Input: part model. Units: mm. Frame: model coordinates. Give positions to 0.01 mm unless a question says otherwise; leave off trailing zeros. Order: outer loops, then holes, each group sorted by start corner. A loop starts at its lowest first (then second) coordinate and runs counter-clockwise, first axis right, second up. Notation, with made-up numbers: (-4, 67.25) - (41, 67.25) arc R14 ccw to (41, 83.25) - close; hole circle Ø10 at (63, -32). An arc over 180 degrees is marked (long way). Use a Markdown table: item, result.
from build123d import *

# Parameters (mm, degrees)
SKETCH1_R                        = 4.951729289
BOSS_EXTRUDE3_DEPTH              = 3
BOSS_EXTRUDE4_DEPTH              = 68
SKETCH5_R                        = 4.5
CUT_EXTRUDE1_DEPTH               = 68
SKETCH11_W                       = 45.01572081
SKETCH11_H                       = 71
CUT_EXTRUDE3_DEPTH               = 2.5
SKETCH12_R                       = 13
BOSS_EXTRUDE7_DEPTH              = 3
SKETCH13_W                       = 45.01572081
SKETCH13_H                       = 71
CUT_EXTRUDE4_DEPTH               = 13
SKETCH14_W                       = 45.01572081
SKETCH14_H                       = 71
BOSS_EXTRUDE8_DEPTH              = 3
SKETCH15_R                       = 1.5
BOSS_EXTRUDE11_DEPTH             = 56.52620135
SKETCH16_R                       = 9
SKETCH16_R_2                     = 4.15
BOSS_EXTRUDE12_DEPTH             = 2
BOSS_EXTRUDE12_DIRECTION_2_REACH = 85.837
SKETCH17_R                       = 9
SKETCH17_R_2                     = 1
BOSS_EXTRUDE13_DEPTH             = 2
SKETCH18_R                       = 13
SKETCH18_R_2                     = 1
BOSS_EXTRUDE14_DEPTH             = 3
SKETCH19_R                       = 1.5
SKETCH19_R_2                     = 1
BOSS_EXTRUDE15_DEPTH             = 56.52620135
CUT_EXTRUDE9_DEPTH               = 43.52620135
SKETCH27_R                       = 10
SKETCH27_R_2                     = 1
CUT_EXTRUDE12_DEPTH              = 10
SKETCH28_R                       = 4.15
CUT_EXTRUDE13_DEPTH              = 73
SKETCH29_R                       = 4.5
SKETCH29_R_2                     = 4.15
CUT_EXTRUDE14_DEPTH              = 73
SKETCH30_R                       = 9
CUT_EXTRUDE15_DEPTH              = 4
SKETCH31_R                       = 10.2
CUT_EXTRUDE17_DEPTH              = 3
CUT_EXTRUDE18_DEPTH              = 197
SKETCH33_W                       = 14.992341928
SKETCH33_H                       = 71
BOSS_EXTRUDE16_DEPTH             = 1
SKETCH34_W                       = 14.992341928
SKETCH34_H                       = 71
BOSS_EXTRUDE17_DEPTH             = 1


with BuildPart() as part:
    # Sketch1 → Boss-Extrude3 (new body)
    with BuildSketch(Plane(origin=(0, 0, 0), x_dir=(1, 0, 0), z_dir=(0, 1, 0))):
        Polygon((-55.988214466, 21.072670098), (19.011785534, 23.055317054), (20.201373708, -21.944682946), (-54.798626292, -23.927329902), align=None)
        with Locations(Location((-17.893420379, -0.436006424, 0), (0, 0, 270))):
            Circle(SKETCH1_R, mode=Mode.SUBTRACT)
    extrude(amount=BOSS_EXTRUDE3_DEPTH)

    # Sketch4 → Boss-Extrude4 (add)
    with BuildSketch(Plane(origin=(0, 3, 0), x_dir=(1, 0, 0), z_dir=(0, 1, 0))):
        Polygon((-54.798626292, -23.927329902), (20.201373708, -21.944682946), (19.011785534, 23.055317054), (-55.988214466, 21.072670098), align=None)
        Polygon((-52.365564518, -21.362137824), (17.636181629, -19.511621172), (16.578723759, 20.490124975), (-53.423022387, 18.639608323), align=None, mode=Mode.SUBTRACT)
    extrude(amount=BOSS_EXTRUDE4_DEPTH)

    # Sketch5 → Cut-Extrude1 (cut)
    with BuildSketch(Plane(origin=(19.607557344, 0, -0.518331518), x_dir=(-0.026426060768931774, 0, -0.9996507706755579), z_dir=(0.999650770675558, 0, -0.026426060768931777))):
        with Locations((0.036998456, 35.5)):
            Circle(SKETCH5_R)
        with BuildLine():
            ThreePointArc((-17.463001544, 29.25), (-19.213001544, 27.5), (-17.463001544, 25.75))
            ThreePointArc((-17.463001544, 25.75), (-15.713001544, 27.5), (-17.463001544, 29.25))
        make_face()
        with BuildLine():
            ThreePointArc((17.536998456, 25.75), (19.286998456, 27.5), (17.536998456, 29.25))
            ThreePointArc((17.536998456, 29.25), (15.786998456, 27.5), (17.536998456, 25.75))
        make_face()
    extrude(amount=-CUT_EXTRUDE1_DEPTH, mode=Mode.SUBTRACT)

    # Sketch11 → Cut-Extrude3 (cut)
    with BuildSketch(Plane(origin=(19.607557344, 0, -0.518331518), x_dir=(-0.026426060768931756, 0, -0.9996507706755579), z_dir=(0.999650770675558, 0, -0.02642606076893176))):
        with Locations((0.036998456, 35.5)):
            Rectangle(SKETCH11_W, SKETCH11_H)
    extrude(amount=-CUT_EXTRUDE3_DEPTH, mode=Mode.SUBTRACT)

    # Sketch12 → Boss-Extrude7 (add)
    with BuildSketch(Plane(origin=(0, 71, 0), x_dir=(1, 0, 0), z_dir=(0, 1, 0))):
        Polygon((17.636181629, -19.511621172), (16.578723759, 20.490124975), (-53.423022387, 18.639608323), (-52.365564518, -21.362137824), align=None)
        with Locations(Location((-17.893420379, -0.436006424, 0), (0, 0, 270))):
            Circle(SKETCH12_R, mode=Mode.SUBTRACT)
    extrude(amount=-BOSS_EXTRUDE7_DEPTH)

    # Sketch13 → Cut-Extrude4 (cut)
    with BuildSketch(Plane(origin=(-55.392442656, 0, 1.464315438), x_dir=(0.02642606076893168, 0, 0.9996507706755579), z_dir=(-0.999650770675558, 0, 0.026426060768931683))):
        with Locations((-0.036998456, 35.5)):
            Rectangle(SKETCH13_W, SKETCH13_H)
    extrude(amount=-CUT_EXTRUDE4_DEPTH, mode=Mode.SUBTRACT)

    # Sketch14 → Boss-Extrude8 (add)
    with BuildSketch(Plane(origin=(-42.396982637, 0, 1.120776648), x_dir=(0.026426060768931694, 0, 0.9996507706755579), z_dir=(-0.999650770675558, 0, 0.026426060768931697))):
        with Locations((-0.036998456, 35.5)):
            Rectangle(SKETCH14_W, SKETCH14_H)
    extrude(amount=-BOSS_EXTRUDE8_DEPTH)

    # Sketch15 → Boss-Extrude11 (add)
    with BuildSketch(Plane(origin=(17.108430418, 0, -0.452266367), x_dir=(-0.02642606076893177, 0, -0.9996507706755579), z_dir=(0.999650770675558, 0, -0.026426060768931774))):
        with BuildLine():
            ThreePointArc((20.044858861, 9.08994731), (14.741558002, 8.303300859), (13.954911551, 3))
            Line((13.954911551, 3), (20.044858861, 3))
            Line((20.044858861, 3), (20.044858861, 9.08994731))
        make_face()
        with Locations((17.923538517, 5.121320344)):
            Circle(SKETCH15_R, mode=Mode.SUBTRACT)
        with BuildLine():
            Line((-19.970861949, 9.08994731), (-19.970861949, 3))
            Line((-19.970861949, 3), (-13.880914639, 3))
            ThreePointArc((-13.880914639, 3), (-14.66756109, 8.303300859), (-19.970861949, 9.08994731))
        make_face()
        with Locations((-17.849541605, 5.121320344)):
            Circle(SKETCH15_R, mode=Mode.SUBTRACT)
        with BuildLine():
            Line((20.044858861, 68), (13.954911551, 68))
            ThreePointArc((13.954911551, 68), (14.741558002, 62.696699141), (20.044858861, 61.91005269))
            Line((20.044858861, 61.91005269), (20.044858861, 68))
        make_face()
        with Locations((17.923538517, 65.878679656)):
            Circle(SKETCH15_R, mode=Mode.SUBTRACT)
        with BuildLine():
            Line((-19.970861949, 68), (-19.970861949, 61.91005269))
            ThreePointArc((-19.970861949, 61.91005269), (-14.66756109, 62.696699141), (-13.880914639, 68))
            Line((-13.880914639, 68), (-19.970861949, 68))
        make_face()
        with Locations((-17.849541605, 65.878679656)):
            Circle(SKETCH15_R, mode=Mode.SUBTRACT)
    extrude(amount=-BOSS_EXTRUDE11_DEPTH)

    # Sketch16 → Boss-Extrude12 (add)
    with BuildSketch(Plane(origin=(0, 3, 0), x_dir=(1, 0, 0), z_dir=(0, 1, 0))):
        with Locations(Location((-17.893420379, -0.436006424, 0), (0, 0, 270))):
            Circle(SKETCH16_R)
        with Locations(Location((-17.893420379, -0.436006424, 0), (0, 0, 270))):
            Circle(SKETCH16_R_2, mode=Mode.SUBTRACT)
    extrude(amount=BOSS_EXTRUDE12_DEPTH)

    # Boss-Extrude12 direction 2: up to this face of the body (flat: up to its plane)
    boss_extrude12_direction_2_end = Plane(part.part.faces().sort_by_distance((-12.489919849, 0, 0.293163306))[0])
    # Sketch16 → Boss-Extrude12 direction 2 (add, up to the picked face)
    with BuildSketch(Plane(origin=(0, 3, 0), x_dir=(1, 0, 0), z_dir=(0, 1, 0)), mode=Mode.PRIVATE) as boss_extrude12_direction_2_sk1:
        with Locations(Location((-17.893420379, -0.436006424, 0), (0, 0, 270))):
            Circle(SKETCH16_R)
        with Locations(Location((-17.893420379, -0.436006424, 0), (0, 0, 270))):
            Circle(SKETCH16_R_2, mode=Mode.SUBTRACT)
    boss_extrude12_direction_2_tool1 = split(extrude(boss_extrude12_direction_2_sk1.sketch, amount=-BOSS_EXTRUDE12_DIRECTION_2_REACH, mode=Mode.PRIVATE), bisect_by=boss_extrude12_direction_2_end, keep=Keep.BOTH, mode=Mode.PRIVATE)
    add(boss_extrude12_direction_2_tool1.solids().sort_by(Axis((-17.89342, 3, -8.309435), (0, -1, 0)))[0])

    # Sketch17 → Boss-Extrude13 (add)
    with BuildSketch(Plane(origin=(0, 5, 0), x_dir=(1, 0, 0), z_dir=(0, 1, 0))):
        with Locations(Location((-17.893420379, -0.436006424, 0), (0, 0, 270))):
            Circle(SKETCH17_R)
        with Locations(Location((-17.893420379, -0.436006424, 0), (0, 0, 270))):
            Circle(SKETCH17_R_2, mode=Mode.SUBTRACT)
    extrude(amount=BOSS_EXTRUDE13_DEPTH)

    # Sketch18 → Boss-Extrude14 (add)
    with BuildSketch(Plane(origin=(0, 71, 0), x_dir=(1, 0, 0), z_dir=(0, 1, 0))):
        with Locations((-17.893420379, -0.436006424)):
            Circle(SKETCH18_R)
        with Locations(Location((-17.893420379, -0.436006424, 0), (0, 0, 270))):
            Circle(SKETCH18_R_2, mode=Mode.SUBTRACT)
    extrude(amount=-BOSS_EXTRUDE14_DEPTH)

    # Sketch19 → Boss-Extrude15 (add)
    with BuildSketch(Plane(origin=(17.108430418, 0, -0.452266367), x_dir=(-0.02642606076893177, 0, -0.9996507706755579), z_dir=(0.999650770675558, 0, -0.026426060768931774))):
        with Locations((-17.849541605, 5.121320344)):
            Circle(SKETCH19_R)
        with Locations((-17.849541605, 5.121320344)):
            Circle(SKETCH19_R_2, mode=Mode.SUBTRACT)
        with Locations((17.923538517, 5.121320344)):
            Circle(SKETCH19_R)
        with Locations((17.923538517, 5.121320344)):
            Circle(SKETCH19_R_2, mode=Mode.SUBTRACT)
        with Locations((-17.849541605, 65.878679656)):
            Circle(SKETCH19_R)
        with Locations((-17.849541605, 65.878679656)):
            Circle(SKETCH19_R_2, mode=Mode.SUBTRACT)
        with Locations((17.923538517, 65.878679656)):
            Circle(SKETCH19_R)
        with Locations((17.923538517, 65.878679656)):
            Circle(SKETCH19_R_2, mode=Mode.SUBTRACT)
    extrude(amount=-BOSS_EXTRUDE15_DEPTH)

    # Sketch23 → Cut-Extrude9 (cut)
    with BuildSketch(Plane(origin=(4.112970399, 0, -0.108727577), x_dir=(-0.02642606076893177, 0, -0.9996507706755579), z_dir=(0.999650770675558, 0, -0.026426060768931774))):
        Polygon((-19.970861949, 68), (-19.970861949, 9.08994731), (-19.970861949, 3), (-13.880914639, 3), (-8.963001544, 3), (-8.963001544, 7), (9.036998456, 7), (9.036998456, 3), (20.044858861, 3), (20.044858861, 9.08994731), (20.044858861, 68), (-13.880914639, 68), align=None)
    extrude(amount=-CUT_EXTRUDE9_DEPTH, mode=Mode.SUBTRACT)

    # Sketch27 → Cut-Extrude12 (cut)
    with BuildSketch(Plane(origin=(0, 71, 0), x_dir=(1, 0, 0), z_dir=(0, 1, 0))):
        with Locations(Location((-17.893420379, -0.436006424, 0), (0, 0, 270))):
            Circle(SKETCH27_R)
        with Locations(Location((-17.893420379, -0.436006424, 0), (0, 0, 270))):
            Circle(SKETCH27_R_2, mode=Mode.SUBTRACT)
    extrude(amount=-CUT_EXTRUDE12_DEPTH, mode=Mode.SUBTRACT)

    # Sketch28 → Cut-Extrude13 (cut)
    with BuildSketch(Plane.XZ):
        with Locations(Location((-17.893420379, 0.436006424, 0), (0, 0, 90))):
            Circle(SKETCH28_R)
    extrude(amount=-CUT_EXTRUDE13_DEPTH, mode=Mode.SUBTRACT)

    # Sketch29 → Cut-Extrude14 (cut)
    with BuildSketch(Plane.XZ):
        with Locations(Location((-17.893420379, 0.436006424, 0), (0, 0, 270))):
            Circle(SKETCH29_R)
        with Locations((-17.893420379, 0.436006424)):
            Circle(SKETCH29_R_2, mode=Mode.SUBTRACT)
    extrude(amount=-CUT_EXTRUDE14_DEPTH, mode=Mode.SUBTRACT)

    # Sketch30 → Cut-Extrude15 (cut)
    with BuildSketch(Plane(origin=(0, 7, 0), x_dir=(1, 0, 0), z_dir=(0, 1, 0))):
        with Locations((-17.893420379, -0.436006424)):
            Circle(SKETCH30_R)
    extrude(amount=-CUT_EXTRUDE15_DEPTH, mode=Mode.SUBTRACT)

    # Sketch31 → Cut-Extrude17 (cut)
    with BuildSketch(Plane(origin=(0, 71, 0), x_dir=(1, 0, 0), z_dir=(0, 1, 0))):
        with Locations(Location((-17.893420379, -0.436006424, 0), (0, 0, 270))):
            Circle(SKETCH31_R)
    extrude(amount=-CUT_EXTRUDE17_DEPTH, mode=Mode.SUBTRACT)

    # Sketch32 → Cut-Extrude18 (cut)
    with BuildSketch(Plane(origin=(0, 71, 0), x_dir=(1, 0, 0), z_dir=(0, 1, 0))):
        Polygon((-42.992754447, 21.416208888), (-42.703678037, 10.480963623), (-32.74415639, 21.687133577), align=None)
        Polygon((-31.554568217, -23.312866423), (-42.092242683, -12.648545848), (-41.803166274, -23.583791112), align=None)
    extrude(amount=-CUT_EXTRUDE18_DEPTH, mode=Mode.SUBTRACT)

    # Sketch33 → Boss-Extrude16 (add)
    with BuildSketch(Plane(origin=(-27.621364057, 0, 27.293341448), x_dir=(0.7028704732937463, 0, 0.7113178598712571), z_dir=(-0.7113178598712571, 0, 0.7028704732937463))):
        with Locations((-13.09208701, 35.5)):
            Rectangle(SKETCH33_W, SKETCH33_H)
    extrude(amount=-BOSS_EXTRUDE16_DEPTH)

    # Sketch34 → Boss-Extrude17 (add)
    with BuildSketch(Plane(origin=(-29.062615571, 0, -25.829498399), x_dir=(-0.6643072639922937, 0, 0.7474596035954538), z_dir=(-0.7474596035954538, 0, -0.6643072639922937))):
        with Locations((13.038095641, 35.5)):
            Rectangle(SKETCH34_W, SKETCH34_H)
    extrude(amount=-BOSS_EXTRUDE17_DEPTH)


solid = part.part
1. Section query B-B (x = -4.5). Return loops of the section in (y, z), then the cut area to 3 significant figures.
Response:
| item | result |
|---|---|
| outline | (0, -22.43) - (71, -22.43) - (71, 22.6) - (0, 22.6) - close; hole (3, -19.93) - (68, -19.93) - (68, 20.1) - (3, 20.1) - close |
| area | 595 mm^2 |
2. Pin query (flat end, axial travel): pin 1 (8 mm diameter, centred on y = 57, z = -7.5, fed in from +X); pin 2 (1 mm diameter, centred on y = 35, z = 18.5, fed in from +X); pin 3 (3 mm diameter, centred on x = -8.5, y = 59, fed in from -Z); pin 4 (1.5 mm diameter, centred on x = -27, z = -4, fed in from +Y). Return the tip coordinate at first contact, or that it passes through.
Response:
| item | result |
|---|---|
| pin 1 | stops at x = -39.52 |
| pin 2 | stops at x = -34.41 |
| pin 3 | stops at z = -22.37 |
| pin 4 | stops at y = 71 |
3. Mould query, pull axis Y, two halves, no side actions, for faces 1 (the face through (-35.865, 35.955, 17.528)), 2 (the face through (-22.286, 1.479, 1.412)). Classes: pulls with the +Y half, pulls with the -Y half, needs draft (parallel to the pull), parting line crosses it, or undercut.
Response:
| item | result |
|---|---|
| face 1 | undercut |
| face 2 | needs draft |
4. Section query A-A (z = 2). Return loops of the section in (x, y), then the cut area to 3 significant figures.
Response:
| item | result |
|---|---|
| outline | (-42.37, 0) - (-22.11, 0) - (-22.11, 3) - (-39.37, 3) - (-39.37, 68) - (-27.97, 68) - (-27.97, 71) - (-42.37, 71) - close; (-13.67, 0) - (17.17, 0) - (17.17, 3) - (-13.67, 3) - close; (-7.81, 68) - (17.17, 68) - (17.17, 71) - (-7.81, 71) - close |
| area | 467 mm^2 |
5. Material intervals for line 1 along Y through (x, z) = (-13.5, 19); line 2 along Y through (x, z) = (15.5, -18.5); line 3 along Z through (x, y) = (14.5, 27.5), sorted ascending.
Response:
| item | result |
|---|---|
| line 1 | y = 0 to 3, 68 to 71 |
| line 2 | y = 0 to 4.13, 6.11 to 9.62, 61.38 to 64.89, 66.87 to 71 |
| line 3 | z = -22.94 to -20.44, 19.59 to 22.1 |
6. Section query C-C (z = -5). Return loops of the section in (x, y).
Response:
| item | result |
|---|---|
| outline | (-42.56, 0) - (16.99, 0) - (16.99, 3) - (-39.56, 3) - (-39.56, 68) - (-26.52, 68) - (-26.52, 71) - (-42.56, 71) - close; (-9.26, 68) - (16.99, 68) - (16.99, 71) - (-9.26, 71) - close |
7. Section query D-D (y = 13.5). Return loops of the section in (x, z), then the cut area to 3 significant figures.
Response:
| item | result |
|---|---|
| outline | (-42.7, -10.48) - (-32.74, -21.69) - (16.51, -22.99) - (16.58, -20.49) - (-33.65, -19.16) - (-39.75, -12.3) - (-39.05, 14.31) - (-32.59, 20.84) - (17.64, 19.51) - (17.7, 22.01) - (-31.55, 23.31) - (-42.09, 12.65) - close |
| area | 348 mm^2 |
